from build123d import *


with BuildPart() as part:
    # Body: sweep along a path in PathSke
    with BuildLine(Plane(origin=(1.207969362, 1.807969362, 0), x_dir=(0, 1, 0), z_dir=(0, 0, 1))) as body_path:
        Line((-0.907969362, -16.792030638), (-0.907969362, -2.792030638))
        ThreePointArc((-0.907969362, -2.792030638), (-0.808285009, -2.285083328), (-0.524075557, -1.853623558))
        ThreePointArc((-0.524075557, -1.853623558), (-1.807969362, 1.207969362), (-3.091863167, -1.853623558))
        ThreePointArc((-3.091863167, -1.853623558), (-2.807653715, -2.285083328), (-2.707969362, -2.792030638))
        Line((-2.707969362, -2.792030638), (-2.707969362, -19.292030638))
    # SectionSke → Body (sweep)
    with BuildSketch(Plane(origin=(18, 0.15, 0.15), x_dir=(0, 1, 0), z_dir=(1, 0, 0))):
        with BuildLine():
            Line((-0.15, -1.05), (-0.15, 0.75))
            ThreePointArc((-0.15, 0.75), (0.75, -0.15), (-0.15, -1.05))
        make_face()
    sweep(path=body_path.line)


solid = part.part
The listing builds one solid part. Answer for the finished solid, in the listing's coordinates (mm). A direction names the side the tool comes from. Round coordinates to 2 decimals unless told otherwise and drop trailing zeros. Order: outer loops, then holes, each group sorted by start corner. A loop starts at its lowest first (then second) coordinate and runs counter-clockwise, first axis right, second up. Notation, with made-up numbers: (-22.5, -34) -> (29.5, -34) arc R26 cw to (29.5, -10) -> close; hole circle Ø2 at (10.5, -23). An arc over 180 degrees is marked (long way). Put each result on its own line as item: value.
Q1. Which of the six approach directions +Z, -Z, +X, -X, +Y, -Y give full straight-line access (tool end or side, diameter ignored) to faces 1 (the flat face through (18, 0.3, 0)), 2 (the flat face through (20.5, -0.4, 0))?
Results list:
face 1: +Z, -Z, +X, +Y
face 2: +Z, -Z, +X, +Y, -Y
Q2. Determine the mould class of faces 3 (the cylindrical face through (3.164, 0.162, -0.013)), 4 (the cylindrical face through (12.4, -0.9, 0)), 5 (the cylindrical face through (10.9, 0.9, 0)) for opening direction Y: pulls with the +Y half, pulls with the -Y half, needs draft (parallel to the pull), parting line crosses it, or undercut.
Results list:
face 3: undercut
face 4: pulls with the -Y half
face 5: pulls with the +Y half
Q3. This flat-tipped pin is pushed along its axis until it touches: P1, Ø0.5, axis at x = 9, z = 0, coming from the +Y side. Where does it stop, or does it pass through?
Results list:
P1: y = 0.9
Q4. Consider line 1 along X through (y, z) = (0.35, 0.4). Determine where the line is inside the solid, lowest interval first.
Results list:
line 1: 0.13 to 0.97, 2.8 to 18
Q5. Section B-B, the plane x = 15.25 is taken. Write down the section's boundary in (y, z).
Results list:
outline: circle Ø1.8 at (0, 0)
